Source: CAD feature listing. Evaluate the final solid. Frame: model axes, mm. A direction names the side the tool comes from. Give positions to 0.01 mm unless a question says otherwise; leave off trailing zeros. Loops run counter-clockwise (first coordinate to the right, second up) from the corner with the lowest first, then second, coordinate; pieces in that order, holes last. Notation, with made-up numbers: (45.25, 64.25) -> (68.25, 64.25) arc R24 cw to (68.25, 79.25) -> close; hole circle Ø5 at (78.25, 81). An arc over 180 degrees is marked (long way). Return JSON: item names as keys, results as strings. Group by question number.
```python
from build123d import *

# Parameters (mm, degrees)
F0_R          = 4.75
F0_R_2        = 2.125
F0_R_3        = 4.25
F1_DEPTH      = 5
F2_W          = 25
F2_H          = 5
F3_DEPTH      = 25
F4_R          = 8.75
F4_R_2        = 4.75
F4_R_3        = 8.25
F4_R_4        = 4.25
F5_DEPTH      = 10
F6_R          = 2.125
F7_DEPTH      = 5.001
F8_W          = 5
F8_H          = 16.9930609057
F8_W_2        = 4
F8_H_2        = 13.3875096302
F9_DEPTH      = 10
F10_T1_DEPTH  = 5
F10_T3_DEPTH  = 4
F10_T8_DEPTH  = 30.7168298797
F10_T13_DEPTH = 29.7168298797
F10_T18_DEPTH = 25.9731600242
F10_S20_R     = 4.75
F10_T21_DEPTH = 15
F10_T25_DEPTH = 13.3875096302


# Not quite as in the source:
# - a fillet or chamfer that OpenCascade refuses, or shapes differently, is made with other operations: its cross-section is extruded or revolved along the edge and cut away or added


with BuildPart() as f1:
    # F0 (on Top) → F1 (new body)
    with BuildSketch(Plane.XY):
        with BuildLine():
            Line((12.5, 26.5), (0, 26.5))
            Line((0, 26.5), (-12.5, 26.5))
            Line((-12.5, 26.5), (-12.5, 8.75))
            ThreePointArc((-12.5, 8.75), (-21.25, 0), (-12.5, -8.75))
            Line((-12.5, -8.75), (-7.5, -8.75))
            Line((-7.5, -8.75), (-7.5, -13.6))
            ThreePointArc((-7.5, -13.6), (-5.3033008589, -18.9033008589), (0, -21.1))
            ThreePointArc((0, -21.1), (5.3033008589, -18.9033008589), (7.5, -13.6))
            Line((7.5, -13.6), (7.5, -8.25))
            ThreePointArc((7.5, -8.25), (15.3166703137, -2.6385915194), (12.5, 6.5622023742))
            Line((12.5, 6.5622023742), (12.5, 26.5))
        make_face()
        with Locations((-12.5, 0)):
            Circle(F0_R, mode=Mode.SUBTRACT)
        with Locations((0, -13.6)):
            Circle(F0_R_2, mode=Mode.SUBTRACT)
        with Locations((7.5, 0)):
            Circle(F0_R_3, mode=Mode.SUBTRACT)
        with Locations((0, 16.5)):
            Circle(F0_R_2, mode=Mode.SUBTRACT)
    extrude(amount=F1_DEPTH)

    # F2 (on face) → F3 (join)
    with BuildSketch(Plane.XY.offset(5)):
        with Locations((0, 24)):
            Rectangle(F2_W, F2_H)
    extrude(amount=F3_DEPTH)

    # F4 (on face) → F5 (join)
    with BuildSketch(Plane.XY.offset(5)):
        with Locations((-12.5, 0)):
            Circle(F4_R)
        with Locations((-12.5, 0)):
            Circle(F4_R_2, mode=Mode.SUBTRACT)
        with Locations((7.5, 0)):
            Circle(F4_R_3)
        with Locations((7.5, 0)):
            Circle(F4_R_4, mode=Mode.SUBTRACT)
    extrude(amount=F5_DEPTH)

    # F6 (on face) → F7 (cut, through all)
    with BuildSketch(Plane.XZ.offset(-21.5)):
        with Locations((0, 22.5)):
            Circle(F6_R)
    extrude(amount=-F7_DEPTH, mode=Mode.SUBTRACT)

    # F8 (on face) → F9 (join)
    with BuildSketch(Plane.XY.offset(5)):
        with Locations((-7.5, 13.0034695472)):
            Rectangle(F8_W, F8_H)
        with Locations((8, 14.8062451849)):
            Rectangle(F8_W_2, F8_H_2)
    extrude(amount=F9_DEPTH)

    # F10: chamfer of 5 on 4 edges, made by hand

    # F10_s2 → F10_t1 (join)
    with BuildSketch(Plane.YZ.offset(-10)):
        Polygon((16.5, 15), (21.5, 20), (21.5, 15), align=None)
    extrude(amount=F10_T1_DEPTH)

    # F10_s4 → F10_t3 (join)
    with BuildSketch(Plane.YZ.offset(6)):
        Polygon((21.5, 20), (16.5, 15), (21.5, 15), align=None)
    extrude(amount=F10_T3_DEPTH)


with BuildPart() as f10_tool6:
    # F10_s7 → F10_t8 (new body)
    with BuildSketch(Plane.YZ.offset(7.8584149398)):
        Polygon((16.5, 15), (21.5, 20), (21.5, 15), align=None)
    extrude(amount=-F10_T8_DEPTH)

    split(bisect_by=Plane.YZ.offset(6), keep=Keep.TOP)


with BuildPart() as f1_1:
    add(f1.part)

    # F10_t5: union F10_tool6
    add(f10_tool6.part)


with BuildPart() as f10_tool11:
    # F10_s12 → F10_t13 (new body)
    with BuildSketch(Plane.YZ.offset(22.8584149398)):
        Polygon((21.5, 20), (16.5, 15), (21.5, 15), align=None)
    extrude(amount=-F10_T13_DEPTH)

    split(bisect_by=Plane.YZ.offset(-5), keep=Keep.BOTTOM)


with BuildPart() as f1_2:
    add(f1_1.part)

    # F10_t10: union F10_tool11
    add(f10_tool11.part)


with BuildPart() as f10_tool16:
    # F10_s17 → F10_t18 (new body)
    with BuildSketch(Plane.XZ.offset(-21.5)):
        Polygon((-10, 10), (-15, 5), (-10, 5), align=None)
    extrude(amount=F10_T18_DEPTH)

    split(bisect_by=Plane.YZ.offset(-12.5), keep=Keep.TOP)

    # F10_s20 → F10_t21 (cut, symmetric)
    with BuildSketch(Plane.XY.offset(7.5)):
        with Locations((-12.5, 0)):
            Circle(F10_S20_R)
    extrude(amount=F10_T21_DEPTH, both=True, mode=Mode.SUBTRACT)


with BuildPart() as f1_3:
    add(f1_2.part)

    # F10_t15: union F10_tool16
    add(f10_tool16.part)


with BuildPart() as f10_tool23:
    # F10_s24 → F10_t25 (new body)
    with BuildSketch(Plane.XZ.offset(-8.1124903698)):
        Polygon((10, 10), (15, 5), (10, 5), align=None)
    extrude(amount=-F10_T25_DEPTH)

    split(bisect_by=Plane.YZ.offset(12.5), keep=Keep.BOTTOM)


with BuildPart() as f1_4:
    add(f1_3.part)

    # F10_t22: union F10_tool23
    add(f10_tool23.part)


solid = f1_4.part
```
1) Cut plane C-C on x = 0. Return loops of the section in (y, z) (3 decimals), then the cut area to 3 significant figures.
2) Reachability of faces 5 (the face through (0, 21.5, 20)), 6 (the face through (-12.5, 23, 9)), 7 (the face through (8, 19, 17.5)), 8 (the face through (12.5, 23, 12)) from +Z, -Z, +X, -X, +Y, -Y: full face, straight path, thin tool, end or side. Return the list, or none.
3) Cut plane B-B on z = 13.25. Return loops of the section in (x, y), then the cut area to 3 significant figures.
4) Mould query, pull axis Y, two halves, no side actions, for faces 1 (the face through (11, 15, 9)), 2 (the face through (0, 26.5, 15)), 3 (the face through (7.5, -11, 2)), 4 (the face through (-10, -8.75, 2)). Classes: released by +Y, released by -Y, zero draft, split by the parting line, or undercut.
5) Material intervals for line 1 (Y direction, x = 0, z = 2.15) (3 decimals); line 2 (X direction, y = 11, z = 12.25); line 3 (Z direction, x = -8.5, y = 12), sorted ascending.
6) Contact query for flat-ended pins moving along their axis: P1, Ø5.5, axis at y = -12, z = 1.5, coming from the -X side; P2, Ø3, axis at y = 14.5, z = 13.5, coming from the +X side; P3, Ø4, axis at x = -10, y = 1, coming from the -Z side; P4, Ø3, axis at x = -3.5, y = -8.5, coming from the +Z side. Output: stop coordinate, or through.
7) Cut plane A-A on z = 22.5. Return loops of the section in (x, y) (3 decimals), then the cut area to 3 significant figures.
8) Cut plane D-D on y = 10.5. Return loops of the section in (x, z).
Calculated:
{
 "1": {"outline": "(-21.1, 0) -> (-15.725, 0) -> (-15.725, 5) -> (-21.1, 5) -> close; (-11.475, 0) -> (14.375, 0) -> (14.375, 5) -> (3.437, 5) -> (3.437, 15) -> (-3.437, 15) -> (-3.437, 5) -> (-11.475, 5) -> close; (18.625, 0) -> (26.5, 0) -> (26.5, 20.375) -> (21.5, 20.375) -> (21.5, 5) -> (18.625, 5) -> close; (21.5, 24.625) -> (26.5, 24.625) -> (26.5, 30) -> (21.5, 30) -> close", "area": "368 mm2"},
 "2": {"face 5": "+Z", "face 6": "+Z, -Z, -X, +Y", "face 7": "+Z, +X, -X, -Y", "face 8": "+Z, -Z, +X, +Y"},
 "3": {"outline": "(-12.5, 21.5) -> (-10, 21.5) -> (-10, 8.39) arc R8.75 ccw (long way) to (-5, 4.51) -> (-5, 21.5) -> (6, 21.5) -> (6, 8.11) arc R8.25 ccw (long way) to (9, 8.11) -> (10, 8.11) -> (10, 21.5) -> (12.5, 21.5) -> (12.5, 26.5) -> (-12.5, 26.5) -> close; hole circle Ø9.5 at (-12.5, 0); hole circle Ø8.5 at (7.5, 0)", "area": "578 mm2"},
 "4": {"face 1": "undercut", "face 2": "released by +Y", "face 3": "zero draft", "face 4": "released by -Y"},
 "5": {"line 1": "-21.1 to -15.725, -11.475 to 14.375, 18.625 to 26.5", "line 2": "-10 to -5, 6 to 10", "line 3": "0 to 15"},
 "6": {"P1": "x = -7.5", "P2": "x = 10", "P3": "through", "P4": "z = 5"},
 "7": {"outline": "(-12.5, 21.5) -> (-2.125, 21.5) -> (-2.125, 26.5) -> (-12.5, 26.5) -> close; (2.125, 21.5) -> (12.5, 21.5) -> (12.5, 26.5) -> (2.125, 26.5) -> close", "area": "104 mm2"},
 "8": {"outline": "(-12.5, 0) -> (12.5, 0) -> (12.5, 7.5) -> (10, 10) -> (10, 15) -> (6, 15) -> (6, 5) -> (-5, 5) -> (-5, 15) -> (-10, 15) -> (-10, 10) -> (-12.5, 7.5) -> close"}
}
